Autodesk Inventor part; units mm, degrees
ref_plane "YZ Plane" through (0, 0, 0) normal (1, 0, 0) x (0, 1, 0)
ref_plane "XZ Plane" through (0, 0, 0) normal (0, 1, 0) x (-1, 0, 0)
ref_plane "XY Plane" through (0, 0, 0) normal (0, 0, 1) x (1, 0, 0)
sketch "Sketch1" plane through (0, 0, 0) normal (0, 1, 0) x (-1, 0, 0)
  point P0 (0, 0)
sketch "Sketch2" plane through (0, 0, 0) normal (0, 1, 0) x (-1, 0, 0)
  point P0 (0, 0)
sketch "Sketch3" plane through (0, 0, 0) normal (0, 1, 0) x (-1, 0, 0)
  circle A0 centre (0, 0) radius 2.25
  line L0 (0, 0) -> (0, 27) construction
  line L1 (0, 27) -> (4.25, 27)
  line L2 (4.25, 27) -> (4.25, -18)
  line L3 (4.25, -18) -> (-4.25, -18)
  line L4 (-4.25, -18) -> (-4.25, 27)
  line L5 (-4.25, 27) -> (0, 27)
  dimension "d0" = 4.5
  dimension "d1" = 27
  dimension "d3" = 45
  dimension "d4" = 8.5
  dimension "d5" = 45
extrude "Extrusion1" add sketch "Sketch3" along normal blind 8
sketch "Sketch4" plane through (0, 8, 0) normal (0, 1, 0) x (1, 0, 0)
  line L0 (-4.25, 18) -> (-4.25, -27)
  line L1 (-4.25, -27) -> (-4.25, -17)
  line L2 (-4.25, -22) -> (-4.25, -17)
  line L3 (-4.25, -17) -> (4.25, -17)
  line L4 (4.25, -27) -> (4.25, 18)
  line L5 (4.25, -27) -> (4.25, -17)
  line L6 (-4.25, -27) -> (4.25, -27)
  point P0 (0, 0)
  dimension "d8" = 10
extrude "Extrusion2" add sketch "Sketch4" along normal blind 30
fillet "Fillet1" radius 4 1 edges at (0, 8, 17)
sketch "Sketch5" plane through (-4.25, 0, 27) normal (0, 0, 1) x (1, 0, 0)
  line L0 (0, 12) -> (0, 38) construction
  line L1 (16.0039, 8) -> (16.0039, 38) construction
  circle A0 centre (4.25, 28) radius 2.25
  line L2 (0, 38) -> (8.5, 38) construction
  line L3 (0, 38) -> (4.25, 38) construction
  line L4 (4.25, 38) -> (4.25, 28) construction
  point P0 (4.25, 0)
  dimension "d12" = 4.5
  dimension "d27" = 4.25
extrude "Extrusion3" cut sketch "Sketch5" against normal blind 20
sketch "Sketch7" plane through (0, 8, 0) normal (0, 1, 0) x (1, 0, 0)
  line L0 (0, 0) -> (0, 13.2) construction
  circle A0 centre (0, 13.2) radius 2.25
  dimension "d18" = 13.2
  dimension "d19" = 4.5
extrude "Extrusion5" cut sketch "Sketch7" against normal blind 19.4625
properties part number "Lconector"
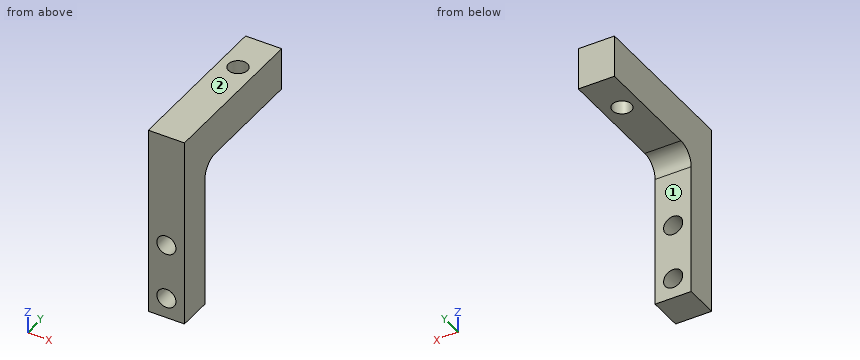
Design review of the part built by this model. Coordinates are the model's own, in mm. Face numbers are marked on the shaded views. A direction names the side the tool comes from. Coordinates: 2 decimals unless noted, no trailing zeros. Loops run counter-clockwise (first coordinate to the right, second up) from the corner with the lowest first, then second, coordinate; pieces in that order, holes last. Notation, with made-up numbers: (79, 63.25) -> (132, 63.25) arc R26 cw to (132, 84.25) -> close; hole circle Ø1 at (36.25, 33.25). An arc over 180 degrees is marked (long way). Use a Markdown table: item, result. Add a question column.
Item 1: Machinability: for the marked faces 1 and 2, which of the approach directions +Z, -Z, +X, -X, +Y, -Y give a long, thin tool a straight path to every point of the face, cutting with its end or side? Answer none if there is none.
Item 2: We need section B-B, the plane z = 0. Write out the cut boundary in (x, y), and give its area (3 significant figures).
Item 3: Clearance check with flat-ended pins moving along their axes: P1, Ø2, axis at x = 0, y = 11, coming from the -Z side; P2, Ø2.5, axis at x = 1, z = -7, coming from the +Y side. State where each tip first meets the part, or that it passes through.
Item 4: We need section D-D, the plane z = 21.5. Write out the cut boundary in (x, y).
Item 5: Wall thickness on L1, parallel to Z at x = 0, y = 6.25; L2, parallel to Z at x = 1.5, y = 5.5; L3, parallel to X at y = 2, z = -13.2: over which ranges is each line inside the solid? List them lowest first. Write a range as from..to.
Item 6: We need section C-C, the plane y = 28. Write out the cut boundary in (x, z), and give its area (3 significant figures).
Item 7: We need section A-A, the plane x = 0. Write out the cut boundary in (y, z), and give its area (3 significant figures).
Numbers:
| question | item | result |
|---|---|---|
| 1 | face 1 | -Z, +X, -X, +Y |
| 1 | face 2 | +Z, +X, -X, +Y, -Y |
| 2 | outline | (-4.25, 0) -> (-2.25, 0) -> (-2.25, 8) -> (-4.25, 8) -> close; (2.25, 0) -> (4.25, 0) -> (4.25, 8) -> (2.25, 8) -> close |
| 2 | area | 32.0 mm^2 |
| 3 | P1 | stops at z = 16.46 |
| 3 | P2 | stops at y = 8 |
| 4 | outline | (-4.25, 0) -> (4.25, 0) -> (4.25, 38) -> (-4.25, 38) -> close; hole circle Ø4.5 at (0, 28) |
| 5 | L1 | z = -18..-15.45, -10.95..-2.25, 2.25..27 |
| 5 | L2 | z = -18..-14.88, -11.52..-1.68, 1.68..27 |
| 5 | L3 | x = -4.25..-2.25, 2.25..4.25 |
| 6 | outline | (-4.25, 17) -> (-2.25, 17) -> (-2.25, 27) -> (-4.25, 27) -> close; (2.25, 17) -> (4.25, 17) -> (4.25, 27) -> (2.25, 27) -> close |
| 6 | area | 40.0 mm^2 |
| 7 | outline | (0, -18) -> (8, -18) -> (8, -15.45) -> (0, -15.45) -> close; (0, -10.95) -> (8, -10.95) -> (8, -2.25) -> (0, -2.25) -> close; (0, 2.25) -> (8, 2.25) -> (8, 13) arc R4 cw to (12, 17) -> (25.75, 17) -> (25.75, 27) -> (0, 27) -> close; (30.25, 17) -> (38, 17) -> (38, 27) -> (30.25, 27) -> close |
| 7 | area | 546 mm^2 |
